Read the model definition and answer for the solid it produces. Units are mm, in the model's axes. Coordinates: 2 decimals unless noted, no trailing zeros. Order: outer loops, then holes, each group sorted by start corner. A loop starts at its lowest first (then second) coordinate and runs counter-clockwise, first axis right, second up. Notation, with made-up numbers: (58, 75) -> (102, 75) arc R30 ccw to (102, 112) -> close; hole circle Ø6 at (42.5, -6). An arc over 180 degrees is marked (long way). Use CSV: the item, a comma, the result in double quotes.
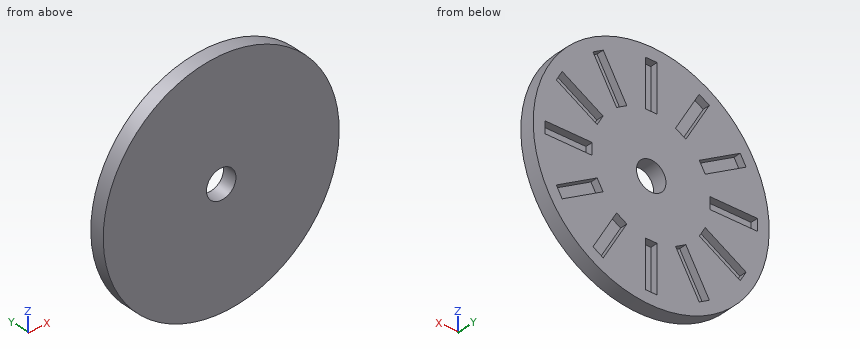
```python
from build123d import *

# Parameters (mm, degrees)
SKETCH1_R               = 101.6
BOSS_EXTRUDE1_DEPTH     = 12.7
CUT_EXTRUDE1_DEPTH      = 6.35
CUT_EXTRUDE2_DEPTH      = 145.244271983
CUT_EXTRUDE2_DEPTH_BACK = 145.244271983
SKETCH3_R               = 12.7


with BuildPart() as part:
    # Sketch1 → Boss-Extrude1 (new body)
    with BuildSketch(Plane(origin=(0, 0, 0), x_dir=(1, 0, 0), z_dir=(0, 1, 0))):
        with Locations(Location((0, 0, 0), (0, 0, 270))):
            Circle(SKETCH1_R)
    extrude(amount=BOSS_EXTRUDE1_DEPTH)

    # Sketch2 → Cut-Extrude1 (cut)
    with BuildSketch(Plane(origin=(0, 12.7, 0), x_dir=(1, 0, 0), z_dir=(0, 1, 0))):
        Polygon((0, 50.8), (5.08, 50.8), (5.08, 91.44), (0, 91.44), (-5.08, 91.44), (-5.08, 50.8), align=None)
        Polygon((25.4, 43.994090512), (29.799409051, 41.454090512), (50.119409051, 76.649362922), (45.72, 79.189362922), (41.320590949, 81.729362922), (21.000590949, 46.534090512), align=None)
        Polygon((43.994090512, 25.4), (46.534090512, 21.000590949), (81.729362922, 41.320590949), (79.189362922, 45.72), (76.649362922, 50.119409051), (41.454090512, 29.799409051), align=None)
        Polygon((50.8, 0), (50.8, -5.08), (91.44, -5.08), (91.44, 0), (91.44, 5.08), (50.8, 5.08), align=None)
        Polygon((43.994090512, -25.4), (41.454090512, -29.799409051), (76.649362922, -50.119409051), (79.189362922, -45.72), (81.729362922, -41.320590949), (46.534090512, -21.000590949), align=None)
        Polygon((25.4, -43.994090512), (21.000590949, -46.534090512), (41.320590949, -81.729362922), (45.72, -79.189362922), (50.119409051, -76.649362922), (29.799409051, -41.454090512), align=None)
        Polygon((0, -50.8), (-5.08, -50.8), (-5.08, -91.44), (0, -91.44), (5.08, -91.44), (5.08, -50.8), align=None)
        Polygon((-25.4, -43.994090512), (-29.799409051, -41.454090512), (-50.119409051, -76.649362922), (-45.72, -79.189362922), (-41.320590949, -81.729362922), (-21.000590949, -46.534090512), align=None)
        Polygon((-43.994090512, -25.4), (-46.534090512, -21.000590949), (-81.729362922, -41.320590949), (-79.189362922, -45.72), (-76.649362922, -50.119409051), (-41.454090512, -29.799409051), align=None)
        Polygon((-50.8, 0), (-50.8, 5.08), (-91.44, 5.08), (-91.44, 0), (-91.44, -5.08), (-50.8, -5.08), align=None)
        Polygon((-43.994090512, 25.4), (-41.454090512, 29.799409051), (-76.649362922, 50.119409051), (-79.189362922, 45.72), (-81.729362922, 41.320590949), (-46.534090512, 21.000590949), align=None)
        Polygon((-25.4, 43.994090512), (-21.000590949, 46.534090512), (-41.320590949, 81.729362922), (-45.72, 79.189362922), (-50.119409051, 76.649362922), (-29.799409051, 41.454090512), align=None)
    extrude(amount=-CUT_EXTRUDE1_DEPTH, mode=Mode.SUBTRACT)

    # Sketch3 → Cut-Extrude2 (cut, two sides: drawn at the far end of the back side and taken through both)
    with BuildSketch(Plane(origin=(0, 12.7, 0), x_dir=(1, 0, 0), z_dir=(0, 1, 0)).offset(-CUT_EXTRUDE2_DEPTH_BACK)):
        with Locations(Location((0, 0, 0), (0, 0, 270))):
            Circle(SKETCH3_R)
    extrude(amount=CUT_EXTRUDE2_DEPTH + CUT_EXTRUDE2_DEPTH_BACK, mode=Mode.SUBTRACT)


solid = part.part
```
Item 1: Find section D-D, the plane x = 27. Give the vertices of the cut face in (y, z).
Return value:
outline,"(0, -97.95) -> (12.7, -97.95) -> (12.7, -56.93) -> (6.35, -56.93) -> (6.35, -43.07) -> (12.7, -43.07) -> (12.7, 43.07) -> (6.35, 43.07) -> (6.35, 56.93) -> (12.7, 56.93) -> (12.7, 97.95) -> (0, 97.95) -> close"
Item 2: Each of these flat-tipped pins is pushed along its axis until it touches: P1, Ø7, axis at x = 1, y = 10, coming from the -Z side; P2, Ø5, axis at x = -66, y = 9, coming from the +Z side; P3, Ø7, axis at x = 68, y = 9.5, coming from the +Z side; P4, Ø1.5, axis at y = 4.5, z = -49, coming from the +X side. Where does it stop, or does it pass through?
Return value:
P1,"stops at z = -101.6"
P2,"stops at z = 79.31"
P3,"stops at z = 78.5"
P4,"stops at x = 89.41"
Item 3: Find section C-C, the plane y = 8.5. Give the number of separate pieces and of enclosed holes in the cut face, then the cut area to 3 significant figures.
Return value:
separate pieces,"1"
enclosed holes,"13"
area,"27,000 mm^2"
Item 4: Find section A-A, the plane x = 0. Give the vertices of the cut face in (y, z).
Return value:
outline,"(0, -101.6) -> (12.7, -101.6) -> (12.7, -91.44) -> (6.35, -91.44) -> (6.35, -50.8) -> (12.7, -50.8) -> (12.7, -12.7) -> (0, -12.7) -> close; (0, 12.7) -> (12.7, 12.7) -> (12.7, 50.8) -> (6.35, 50.8) -> (6.35, 91.44) -> (12.7, 91.44) -> (12.7, 101.6) -> (0, 101.6) -> close"
Item 5: Find section B-B, the plane z = 0. Give the vertices of the cut face in (x, y).
Return value:
outline,"(-101.6, 0) -> (-12.7, 0) -> (-12.7, 12.7) -> (-50.8, 12.7) -> (-50.8, 6.35) -> (-91.44, 6.35) -> (-91.44, 12.7) -> (-101.6, 12.7) -> close; (12.7, 0) -> (101.6, 0) -> (101.6, 12.7) -> (91.44, 12.7) -> (91.44, 6.35) -> (50.8, 6.35) -> (50.8, 12.7) -> (12.7, 12.7) -> close"
Item 6: Straight lines are drawn through the part: line 1 along X through (y, z) = (7.5, 0); line 2 along X through (y, z) = (9.5, 51); line 3 along Z through (x, y) = (64.5, 7.5). For each, find the intervals that lie inside material, in ascending order.
Return value:
line 1,"x = -101.6 to -91.44, -50.8 to -12.7, 12.7 to 50.8, 91.44 to 101.6"
line 2,"x = -87.87 to -35.31, -23.58 to -5.08, 5.08 to 23.58, 35.31 to 87.87"
line 3,"z = -78.5 to -43.1, -31.37 to -5.08, 5.08 to 31.37, 43.1 to 78.5"
